from build123d import *

# Parameters (mm, degrees)
F0_R     = 70.413899
F1_DEPTH = 5
F2_R     = 15.708766
F3_DEPTH = 5.001
F4_COUNT = 6
F4_ANGLE = 200


with BuildPart() as f1:
    # F0 (on Top) → F1 (new body)
    with BuildSketch(Plane.XY):
        Circle(F0_R)
    extrude(amount=F1_DEPTH)

    # F2 (on face) → F3 (cut, through all)
    with BuildSketch(Plane.XY.offset(5)):
        with Locations((-30.731812, -27.514353)):
            Circle(F2_R)
    extrude(amount=-F3_DEPTH, mode=Mode.SUBTRACT)

    # F4: F1 ×6 about axis
    f4_axis = Axis((-30.731812, -27.514353, 0), (0, 0, 1))


with BuildPart() as f1_1:
    add(f1.part)
    for i in range(1, F4_COUNT):
        add(f1.part.rotate(f4_axis, i * F4_ANGLE / (F4_COUNT - 1)))


solid = f1_1.part
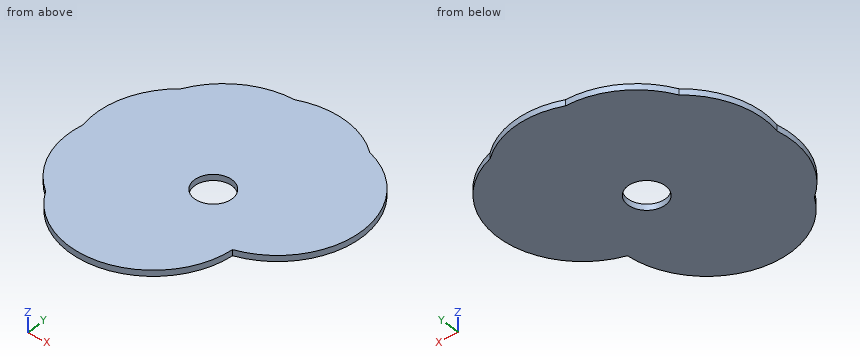
Build history of the part. All positions in model axes, mm. Round coordinates to 2 decimals unless told otherwise and drop trailing zeros. Write each loop counter-clockwise with the first axis right and the second up, starting at its lowest first coordinate (ties: lowest second). Pieces come first, ordered by that corner, then holes. Notation, with made-up numbers: (9, 81) -> (64, 81) arc R37 ccw to (64, 118) -> close; hole circle Ø8 at (35.25, -38). An arc over 180 degrees is marked (long way). Use one line per item in the form item = value.
Q1. Band-saw the part on B-B, the plane y = -36. Write the cut outline in (x, z).
Conclusion:
outline = (-139.1, 0) -> (-43.95, 0) -> (-43.95, 5) -> (-139.1, 5) -> close; (-17.51, 0) -> (60.52, 0) -> (60.52, 5) -> (-17.51, 5) -> close
Q2. Band-saw the part on D-D, the plane y = -58. Write the cut outline in (x, z), then the cut area to 3 significant figures.
Conclusion:
outline = (-137.79, 0) -> (39.93, 0) -> (39.93, 5) -> (-137.79, 5) -> close
area = 889 mm²
Q3. Drop flat-ended pins along their axis: P1, Ø25, axis at x = -30.73, y = -27.51, coming from the +Z side; P2, Ø3, axis at x = 18, z = 4, coming from the +Y side; P3, Ø2, axis at y = -20, z = 4, coming from the -X side; P4, Ø1.5, axis at y = -105.5, z = 1.5, coming from the +X side. Give the stop position or say it passes through.
Conclusion:
P1 = through
P2 = 70.29
P3 = -140.21
P4 = 7.14
Q4. Band-saw the part on C-C, the plane z = 2.3. Write the cut outline in (x, y).
Conclusion:
outline = (-138.42, -30.97) arc R70.41 ccw to (-111.01, -99.39) arc R70.41 ccw to (20.12, -67.48) arc R70.41 ccw to (20.12, 67.48) arc R70.41 ccw to (-52.84, 77.94) arc R70.41 ccw to (-115.45, 39.06) arc R70.41 ccw to start; hole circle Ø31.42 at (-30.73, -27.51)
Q5. Band-saw the part on A-A, the plane x = -37. Write the cut outline in (y, z).
Conclusion:
outline = (-133.05, 0) -> (-41.92, 0) -> (-41.92, 5) -> (-133.05, 5) -> close; (-13.11, 0) -> (82.68, 0) -> (82.68, 5) -> (-13.11, 5) -> close
Q6. Drill centre lines: L1, parallel to Y at x = -31.5, z = 2; L2, parallel to X at y = -32, z = 1.6; L3, parallel to X at y = -17, z = 1.65. Where is each one in solid material? Low to high.
Conclusion:
L1 = -131.77 to -43.2, -11.82 to 83.42
L2 = -138.59 to -45.79, -15.68 to 62.72
L3 = -140.3 to -42.4, -19.06 to 68.33
